Check sheet for the modelled part. Datum: model origin and axes. Units: mm. Give positions to 0.01 mm unless a question says otherwise; leave off trailing zeros. Order: outer loops, then holes, each group sorted by start corner. A loop starts at its lowest first (then second) coordinate and runs counter-clockwise, first axis right, second up.
Autodesk Inventor part; units mm, degrees
ref_plane "YZ Plane" through (0, 0, 0) normal (1, 0, 0) x (0, 1, 0)
ref_plane "XZ Plane" through (0, 0, 0) normal (0, 1, 0) x (-1, 0, 0)
ref_plane "XY Plane" through (0, 0, 0) normal (0, 0, 1) x (1, 0, 0)
sketch "スケッチ1" plane through (0, 0, 0) normal (0, 0, 1) x (1, 0, 0)
  circle A0 centre (0, 0) radius 3
  dimension "d0" = 6
extrude "押し出し1" add sketch "スケッチ1" along normal blind 30
sketch "スケッチ2" plane through (0, 0, 30) normal (0, 0, 1) x (1, 0, 0)
  circle A0 centre (0, 0) radius 1.4
  dimension "d3" = 2.8
extrude "押し出し2" cut sketch "スケッチ2" against normal blind 6
sketch "スケッチ3" plane through (0, 0, 0) normal (0, 0, -1) x (-1, 0, 0)
  circle A0 centre (0, 0) radius 1.4
  circle A1 centre (0, 0) radius 1.4
extrude "押し出し3" cut sketch "スケッチ3" against normal blind 6
properties part number "34mm" material "アルミニウム 6061"
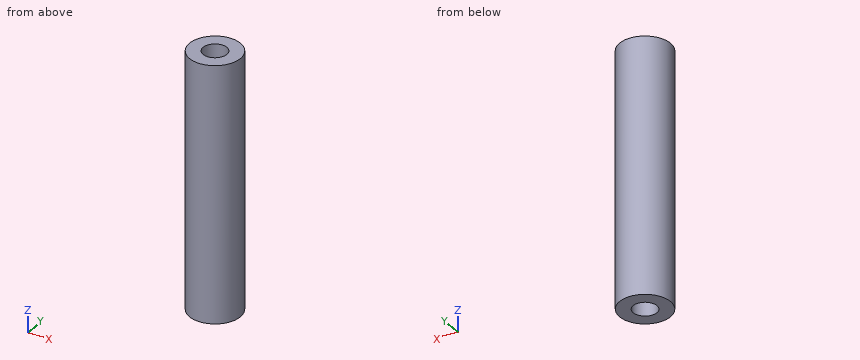
Q1. Material ranges on line 1 (Y direction, x = 0, z = 28.1); line 2 (X direction, y = 1, z = 28); line 3 (Y direction, x = 0.2, z = 20), recorded low to high.
Q2. Sectioned sample at C-C, the plane z = 8. Record the cut outline in (x, y), plus the area to 3 significant figures.
Q3. Sectioned sample at D-D, the plane y = -2.6. Record the cut outline in (x, z), plus the area to 3 significant figures.
Q4. Sectioned sample at A-A, the plane x = 0. Record the cut outline in (y, z).
Q5. Go/stop test with flat-tipped pins: P1, Ø2, axis at x = 0, y = 0, coming from the +Z side; P2, Ø1.5, axis at x = -1.5, z = 26, coming from the -Y side; P3, Ø3, axis at y = 2, z = 18.5, coming from the -X side. Record where each tip stops, or that it passes through.
Filled in:
1. line 1: y = -3 to -1.4, 1.4 to 3
1. line 2: x = -2.83 to -0.98, 0.98 to 2.83
1. line 3: y = -2.99 to 2.99
2. outline: circle Ø6 at (0, 0)
2. area: 28.3 mm2
3. outline: (-1.5, 0) - (1.5, 0) - (1.5, 30) - (-1.5, 30) - close
3. area: 89.8 mm2
4. outline: (-3, 0) - (-1.4, 0) - (-1.4, 6) - (1.4, 6) - (1.4, 0) - (3, 0) - (3, 30) - (1.4, 30) - (1.4, 24) - (-1.4, 24) - (-1.4, 30) - (-3, 30) - close
5. P1: stops at z = 24
5. P2: stops at y = -2.9
5. P3: stops at x = -2.96
